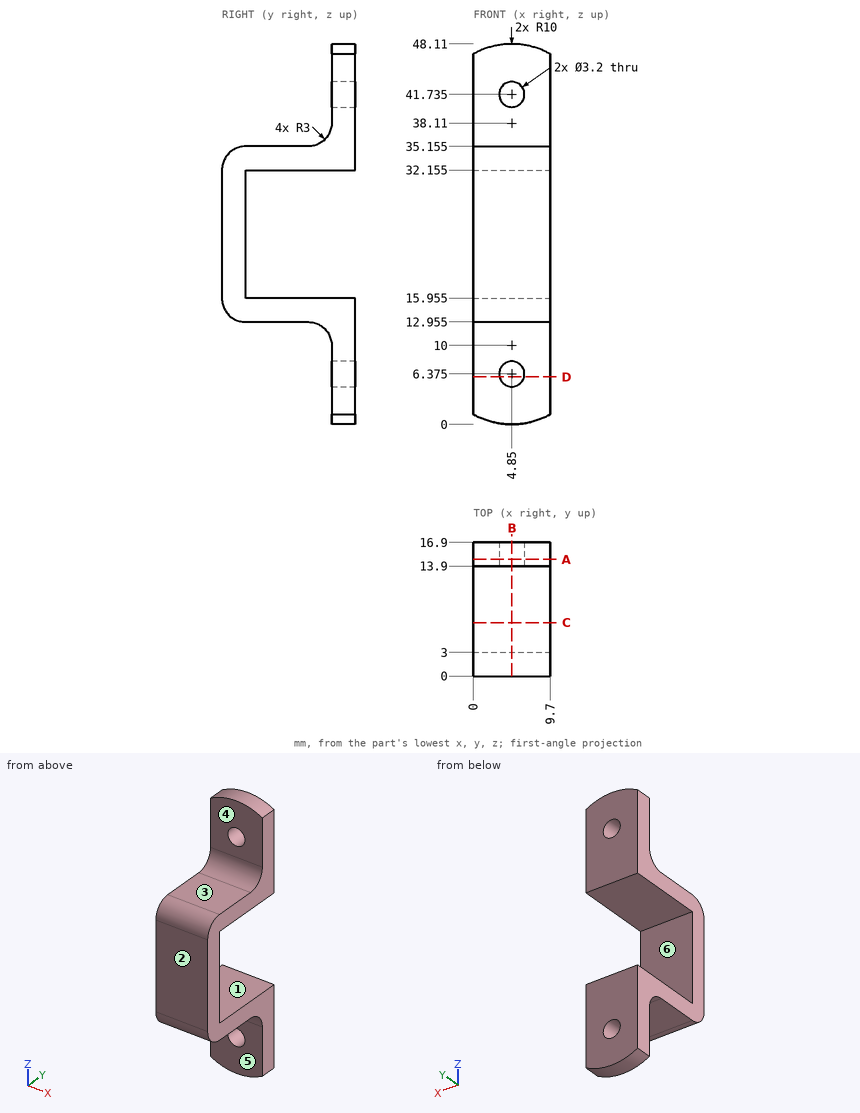
For this review, use the dimensioned drawing (mm, ordinates from the lowest corner) and the shaded views. A direction names the side the tool comes from. Give positions to 0.01 mm unless a question says otherwise; leave off trailing zeros. Write each loop counter-clockwise with the first axis right and the second up, starting at its lowest first coordinate (ties: lowest second). Pieces come first, ordered by that corner, then holes. Notation, with made-up numbers: M 40.25,74.5 L 98.25,74.5 A37 ccw 98.25,110.5 Z; hole C 77.5,77 d6. An arc over 180 degrees is marked long. Write item = value, one per line. Start each with the question number.
Q1. We need section D-D (z = 6). State the section outline as (x, y) points (1 decimal).
Q2. We need section C-C (y = 6.75). State the section outline as (x, z) points (1 decimal), plus the area to 3 significant figures.
Q3. Clearance check with flat-ended pins moving along their axes: pin 1 (5 mm diameter, centred on x = 8.5, y = 7.5, fed in from -Z) (3 decimals); pin 2 (5 mm diameter, centred on x = 2.5, y = 12, fed in from +Z); pin 3 (5 mm diameter, centred on x = 6.5, z = 2.5, fed in from -Y). State where each tip first meets the part, or that it passes through.
Q4. Mouldability with a two-part tool opening along Z and no side actions: class the marked faces 1, 2 and 3 as released by +Z, released by -Z, zero draft, split by the parting line, or undercut.
Q5. We need section A-A (y = 14.75). Give the number of separate pieces and of enclosed holes in the cut face.
Q6. For line 1 (Z direction, x = 4.5, y = 7.25) (1 decimal); line 2 (Z direction, x = 6, y = 15.25) (1 decimal); line 3 (Z direction, x = 7.25, y = 14) (1 decimal), list the stretches that pass through material, from the lowest coordinate up.
Q7. We need section B-B (x = 4.85). State the section outline as (y, z) points (1 decimal).
Q8. Machinability: for the marked faces 4, 5 and 6, which of the approach directions +Z, -Z, +X, -X, +Y, -Y give a long, thin tool a straight path to every point of the face, cutting with its end or side? Answer none if there is none.
Result set:
q1.outline = M 0,13.9 L 3.3,13.9 L 3.3,16.9 L 0,16.9 Z; M 6.4,13.9 L 9.7,13.9 L 9.7,16.9 L 6.4,16.9 Z
q2.outline = M 0,13 L 9.7,13 L 9.7,16 L 0,16 Z; M 0,32.2 L 9.7,32.2 L 9.7,35.2 L 0,35.2 Z
q2.area = 58.2 mm2
q3.pin_1 = 12.955
q3.pin_2 = 48.08
q3.pin_3 = 13.9
q4.face_1 = undercut
q4.face_2 = zero draft
q4.face_3 = released by +Z
q5.separate_pieces = 2
q5.enclosed_holes = 2
q6.line_1 = 13 to 16, 32.2 to 35.2
q6.line_2 = 0.1 to 5.3, 7.5 to 16, 32.2 to 40.6, 42.8 to 48
q6.line_3 = 0.3 to 16, 32.2 to 47.8
q7.outline = M 0,16 A3 ccw 3,13 L 10.9,13 A3 cw 13.9,10 L 13.9,8 L 16.9,8 L 16.9,16 L 3,16 L 3,32.2 L 16.9,32.2 L 16.9,40.1 L 13.9,40.1 L 13.9,38.2 A3 cw 10.9,35.2 L 3,35.2 A3 ccw 0,32.2 Z; M 13.9,0 L 16.9,0 L 16.9,4.8 L 13.9,4.8 Z; M 13.9,43.3 L 16.9,43.3 L 16.9,48.1 L 13.9,48.1 Z
q8.face_4 = +Z, +X, -X, -Y
q8.face_5 = -Z, +X, -X, -Y
q8.face_6 = +X, -X, +Y
